The model under review builds one solid part; all positions refer to its coordinate system, in mm. A direction names the side the tool comes from. Round coordinates to 2 decimals unless told otherwise and drop trailing zeros. Write each loop counter-clockwise with the first axis right and the second up, starting at its lowest first coordinate (ties: lowest second). Pieces come first, ordered by that corner, then holes. Notation, with made-up numbers: (45.5, 38.5) - (72.5, 38.5) arc R34 ccw to (72.5, 68.5) - close; hole circle Ø7 at (24.25, 18.5). An arc over 180 degrees is marked (long way). Return JSON: item names as keys, results as strings.
from build123d import *

# Parameters (mm, degrees)
SKETCH_1_R      = 16
SKETCH_1_R_2    = 12.5
EXTRUDE_1_DEPTH = 35
SKETCH_2_R      = 16
SKETCH_2_R_2    = 12.5
EXTRUDE_2_DEPTH = 35
REVOLVE_1_ANGLE = 90


with BuildPart() as part:
    # 草图1 → 凸台-拉伸1 (new body)
    with BuildSketch(Plane.XY):
        Circle(SKETCH_1_R)
        Circle(SKETCH_1_R_2, mode=Mode.SUBTRACT)
    extrude(amount=EXTRUDE_1_DEPTH)

    # 草图2 → 凸台-拉伸2 (add)
    with BuildSketch(Plane(origin=(0, 0, 0), x_dir=(0, 0, -1), z_dir=(1, 0, 0))):
        Circle(SKETCH_2_R)
        Circle(SKETCH_2_R_2, mode=Mode.SUBTRACT)
    extrude(amount=EXTRUDE_2_DEPTH)

    # 草图3 → 旋转1 (revolve)
    with BuildSketch(Plane.XY):
        with BuildLine():
            Line((0, 16), (0, -16))
            ThreePointArc((0, -16), (-16, 0), (0, 16))
        make_face()
    revolve(axis=Axis((0, 16, 0), (0, -1, 0)), revolution_arc=REVOLVE_1_ANGLE)


solid = part.part
(1) Add section A-A (y = 0). Write out the cut boundary in (x, z), plus the area to 3 significant figures.
Filled in:
{"outline": "(-16, 0) arc R16 ccw to (0, -16) - (35, -16) - (35, -12.5) - (0, -12.5) - (0, 0) - (-12.5, 0) - (-12.5, 35) - (-16, 35) - close; (0, 12.5) - (12.5, 12.5) - (12.5, 0) - (16, 0) - (16, 12.5) - (35, 12.5) - (35, 16) - (16, 16) - (16, 35) - (12.5, 35) - (12.5, 16) - (0, 16) - close", "area": "679 mm2"}
(2) Wall thickness on line 1 (Y direction, x = 0, z = 27.5): over which ranges is the line inside the solid? List them lowest first.
Filled in:
{"line 1": "y = -16 to -12.5, 12.5 to 16"}
(3) For faces 1 (the cylindrical face through (-12.488, 0.55, 21.144)), 2 (the flat face through (0, 0, -5)), 3 (the cylindrical face through (4.774, 0.275, 12.497)), 4 (the flat face through (-10, -8, 35)), list the 3-axis set-ups (+Z, -Z, +X, -X, +Y, -Y) from which the entire face can be reached by the end or side of a thin tool; tool diameter is ignored.
Filled in:
{"face 1": "+Z", "face 2": "+X", "face 3": "none", "face 4": "+Z, +X, -X, +Y, -Y"}
(4) Add section C-C (x = 5.5). Write out the cut boundary in (y, z).
Filled in:
{"outline": "(-15.02, 5.5) arc R16 ccw (long way) to (15.02, 5.5) - (15.02, 35) - (11.22, 35) - (11.22, 11.4) arc R16 ccw to (-11.22, 11.4) - (-11.22, 35) - (-15.02, 35) - close; hole (-12.5, 0) arc R12.5 ccw to (12.5, 0) - (11.22, 0) - (11.22, 5.5) arc R12.5 ccw to (-11.22, 5.5) - (-11.22, 0) - close"}
(5) Mouldability with a two-part tool opening along Y and no side actions: class faces 5 (the flat face through (13, 1, 0)), 6 (the flat face through (35, -8, 10)), 7 (the cylindrical face through (21.14, -6.13, -14.78)) as released by +Y, released by -Y, zero draft, split by the parting line, or undercut.
Filled in:
{"face 5": "undercut", "face 6": "zero draft", "face 7": "split by the parting line"}
(6) Clearance check with flat-ended pins moving along their axes: pin 1 Ø6 at (x, z) = (18, 6) entering from +Y; pin 2 Ø2 at (x, z) = (7, 10) entering from -Y; pin 3 Ø1.5 at (x, y) = (-6, 4) entering from -Z. State where each tip first meets the part, or that it passes through.
Filled in:
{"pin 1": "stops at y = 15.72", "pin 2": "stops at y = -14.83", "pin 3": "stops at z = -14.64"}
(7) Add section D-D (y = 11). Write out the cut boundary in (x, z), plus the area to 3 significant figures.
Filled in:
{"outline": "(-11.62, 0) arc R11.62 ccw to (0, -11.62) - (35, -11.62) - (35, -5.94) - (0, -5.94) - (0, 0) - (-5.94, 0) - (-5.94, 35) - (-11.62, 35) - close; (0, 5.94) - (5.94, 5.94) - (5.94, 0) - (11.62, 0) - (11.62, 5.94) - (35, 5.94) - (35, 11.62) - (11.62, 11.62) - (11.62, 35) - (5.94, 35) - (5.94, 11.62) - (0, 11.62) - close", "area": "869 mm2"}
(8) Add section B-B (z = 8.5). Write out the cut boundary in (x, y).
Filled in:
{"outline": "(8.5, -13.56) - (35, -13.56) - (35, -9.17) - (13.11, -9.17) arc R16 ccw to (13.11, 9.17) - (35, 9.17) - (35, 13.56) - (8.5, 13.56) arc R16 ccw (long way) to start; hole (0, -12.5) - (0, -9.17) - (8.5, -9.17) arc R12.5 ccw to (8.5, 9.17) - (0, 9.17) - (0, 12.5) arc R12.5 ccw to start"}
